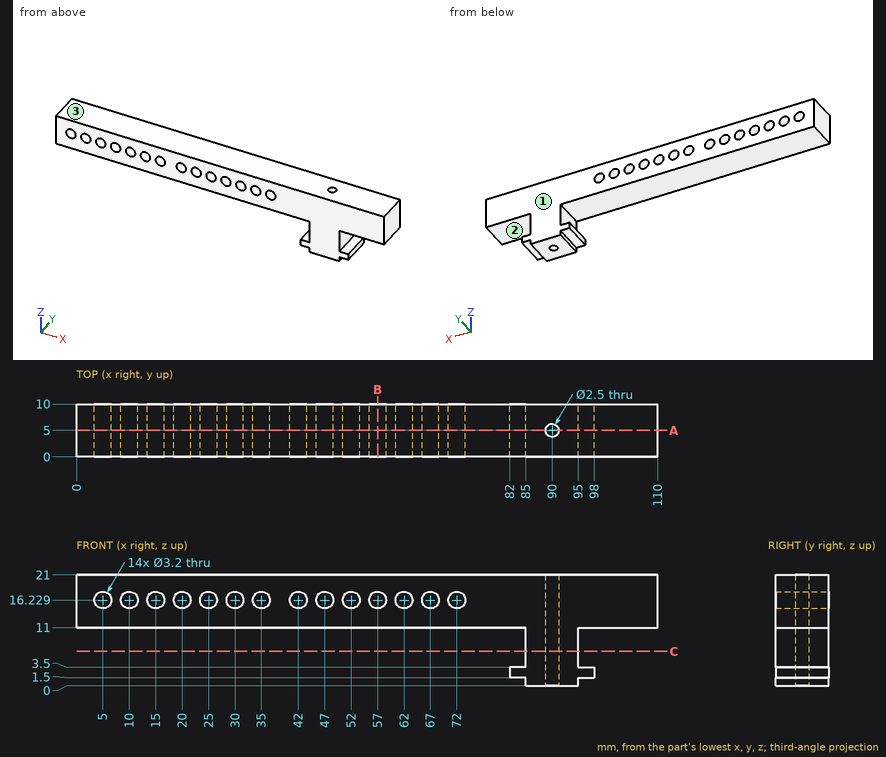
For this review, use the dimensioned drawing (mm, ordinates from the lowest corner) and the shaded views. Coordinates: 2 decimals unless noted, no trailing zeros. Order: outer loops, then holes, each group sorted by start corner. A loop starts at its lowest first (then second) coordinate and runs counter-clockwise, first axis right, second up. Notation, with made-up numbers: (6.25, 41.5) - (43.25, 41.5) arc R6 ccw to (43.25, 46.5) - close; hole circle Ø3 at (-38, 22). An arc over 180 degrees is marked (long way). Answer as a JSON object with one key per item and string values. Group by question number.
1. We need section A-A on y = 5. Give the number of separate pieces and of enclosed holes in the cut face, then the cut area to 3 significant figures.
2. Clearance check with flat-ended pins moving along their axes: P1, Ø12, axis at x = 66.5, z = 3, coming from the -Y side; P2, Ø6, axis at x = 17, y = 2.5, coming from the -Z side; P3, Ø1, axis at y = 5.5, z = 2, coming from the +X side; P4, Ø1.5, axis at y = 5, z = 8, coming from the +X side. State where each tip first meets the part, or that it passes through.
3. For probe 1 along Z at (x, y) = (5, 7.25); probe 2 along Z at (x, y) = (32.5, 9); probe 3 along Z at (x, y) = (63, 3.25), list the stretches that pass through material, from the lowest coordinate up.
4. We need section C-C on z = 6.5. State the section outline as (x, y) points.
5. We need section B-B on x = 57. State the section outline as (y, z) points.
6. The part is to be moulded in two halves that separate along Z. For the marked faces 1, 2 and 3, say which applies: pulls with the +Z half, pulls with the -Z half, needs draft (parallel to the pull), parting line crosses it, or undercut.
Final values:
{
 "1": {"separate pieces": "2", "enclosed holes": "14", "area": "1,060 mm²"},
 "2": {"P1": "through", "P2": "z = 11", "P3": "x = 98", "P4": "x = 95"},
 "3": {"probe 1": "11 to 14.63, 17.83 to 21", "probe 2": "11 to 21", "probe 3": "11 to 14.98, 17.48 to 21"},
 "4": {"outline": "(85, 0) - (95, 0) - (95, 10) - (85, 10) - close; hole circle Ø2.5 at (90, 5)"},
 "5": {"outline": "(0, 11) - (10, 11) - (10, 14.63) - (0, 14.63) - close; (0, 17.83) - (10, 17.83) - (10, 21) - (0, 21) - close"},
 "6": {"face 1": "needs draft", "face 2": "undercut", "face 3": "pulls with the +Z half"}
}
